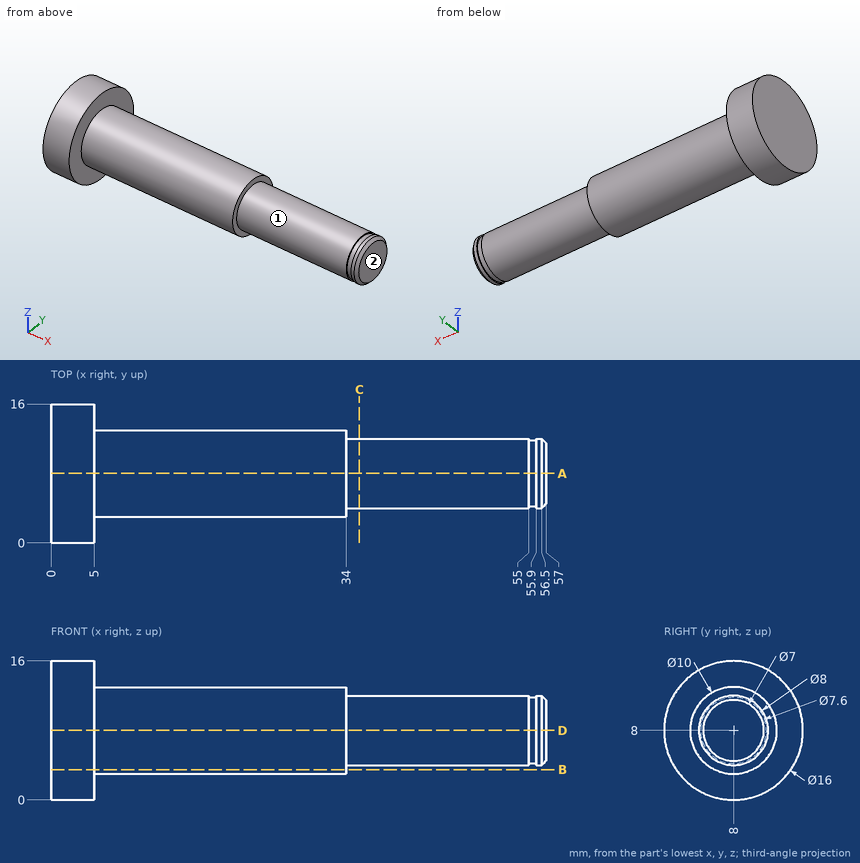
Job drawing, mm, ordinate dimensions from the low corner. One solid piece. A direction names the side the tool comes from. Round coordinates to 2 decimals unless told otherwise and drop trailing zeros. Order: outer loops, then holes, each group sorted by start corner. A loop starts at its lowest first (then second) coordinate and runs counter-clockwise, first axis right, second up. Notation, with made-up numbers: M -35,87.25 L 17,87.25 A29 ccw 17,115.25 Z; hole C 49,35.5 d8. An arc over 180 degrees is marked long. Write each question's results on one line, items separated by ' | '. Start each with the question number.
(1) Drop flat-ended pins along their axis: pin 1 (6 mm diameter, centred on x = 47, y = 6, fed in from -Z); pin 2 (4 mm diameter, centred on x = 49.5, y = 5.5, fed in from +Z); pin 3 (1 mm diameter, centred on x = 46.5, z = 12, fed in from +Y). Give the stop position or say it passes through.
(2) Saw through at B-B, the plane z = 3.5. Give the cut face in (x, y).
(3) Which spindle directions (+Z, -Z, +X, -X, +Y, -Y) get a long thin tool onto all of the face, cutting with end or side? Do the marked faces 1 and 2. Say none if no direction does.
(4) Saw through at A-A, the plane y = 8. Give the cut face in (x, z), then the cut area to 3 significant figures.
(5) Saw through at C-C, the plane x = 35.5. Give the cut face in (y, z).
(6) Probe probe 1 along X at (y, z) = (0.5, 5.5); probe 2 along X at (y, z) = (10, 4.25); probe 3 along Y at (x, z) = (33, 11). List the from-to ranges inside material, lowest first. Write a range as from..to.
Established:
1) pin 1: stops at z = 4 | pin 2: stops at z = 11.97 | pin 3: stops at y = 9.94
2) outline: M 0,1.39 L 5,1.39 L 5,5.82 L 34,5.82 L 34,10.18 L 5,10.18 L 5,14.61 L 0,14.61 Z
3) face 1: +X | face 2: +Z, -Z, +X, +Y, -Y
4) outline: M 0,0 L 5,0 L 5,3 L 34,3 L 34,4 L 55,4 L 55,4.2 L 55.9,4.2 L 55.9,4 L 56.5,4 L 57,4.5 L 57,11.5 L 56.5,12 L 55.9,12 L 55.9,11.8 L 55,11.8 L 55,12 L 34,12 L 34,13 L 5,13 L 5,16 L 0,16 Z | area: 553 mm^2
5) outline: C 8,8 d8
6) probe 1: x = 0..5 | probe 2: x = 0..34 | probe 3: y = 4..12
